from build123d import *
from OCP.BRepFilletAPI import BRepFilletAPI_MakeChamfer

# Parameters (mm, degrees)
EXTRUDE_1_DEPTH                     = 8.5
SKETCH_4_W                          = 0.7
SKETCH_4_H                          = 0.7
CUT_EXTRUDE_1_DEPTH                 = 8.2
CHAMFER_3_SIZE                      = 0.4
SKETCH_2_W                          = 0.4
SKETCH_2_H                          = 0.6
EXTRUDE_2_DEPTH                     = 3
CHAMFER_2_SIZE                      = 0.5
CHAMFER_2_SIZE2                     = 0.106278281
PATTERN_LINEAR_1_COUNT              = 3
PATTERN_LINEAR_1_PITCH              = 2.54
PATTERN_LINEAR_1_COUNT_DIR2         = 2
PATTERN_LINEAR_1_PITCH_DIR2         = 2.54
CHAMFER_3_OF_PATTERN_LINEAR_1_SIZE  = 0.4
CHAMFER_2_OF_PATTERN_LINEAR_1_SIZE  = 0.5
CHAMFER_2_OF_PATTERN_LINEAR_1_SIZE2 = 0.106278281


with BuildPart() as part:
    # Эскиз1 → Бобышка-Вытянуть1 (new body)
    with BuildSketch(Plane(origin=(0, 0, 0), x_dir=(-1, 0, 0), z_dir=(0, 1, 0))):
        Polygon((-1.27, 1.52), (1.27, 1.52), (3.81, 1.52), (3.81, -1.52), (3.81, -6.6), (-1.27, -6.6), (-1.27, -1.52), align=None)
    extrude(amount=EXTRUDE_1_DEPTH)

    # Эскиз4 → Вырез-Вытянуть1 (cut)
    with BuildSketch(Plane(origin=(0, 8.5, 0), x_dir=(1, 0, 0), z_dir=(0, 1, 0))):
        Rectangle(SKETCH_4_W, SKETCH_4_H)
    cut_extrude_1 = extrude(amount=-CUT_EXTRUDE_1_DEPTH, mode=Mode.SUBTRACT)

    # Фаска3
    chamfer_3_edges = [part.edges().sort_by_distance(p)[0] for p in [
        (-0.35, 8.5, 0),
        (0, 8.5, 0.35),
        (0.35, 8.5, 0),
        (0, 8.5, -0.35),
    ]]
    chamfer(chamfer_3_edges, length=CHAMFER_3_SIZE)

    # Эскиз2 → Бобышка-Вытянуть2 (add)
    with BuildSketch(Plane(origin=(0, 0, 0), x_dir=(-1, 0, 0), z_dir=(0, 1, 0))):
        Rectangle(SKETCH_2_W, SKETCH_2_H)
    extrude_2 = extrude(amount=-EXTRUDE_2_DEPTH)

    # Фаска2: one chamfer whose edges measure the first distance from different faces: ONE call of the kernel's chamfer builder (chamfer() names one face for all edges)
    chamfer_2_edges_1 = [part.edges().sort_by_distance(p)[0] for p in [
        (-0.2, -3, 0),
    ]]
    chamfer_2_side_1 = [part.faces().sort_by_distance(p)[0] for p in [
        (-0.2, -1.5, 0),
    ]]
    chamfer_2_edges_2 = [part.edges().sort_by_distance(p)[0] for p in [
        (0.2, -3, 0),
    ]]
    chamfer_2_side_2 = [part.faces().sort_by_distance(p)[0] for p in [
        (0.2, -1.5, 0),
    ]]
    chamfer_2 = BRepFilletAPI_MakeChamfer(part.part.solid().wrapped)
    for e in chamfer_2_edges_1:
        chamfer_2.Add(CHAMFER_2_SIZE, CHAMFER_2_SIZE2, e.wrapped, chamfer_2_side_1[0].wrapped)  # the first distance lies on this face
    for e in chamfer_2_edges_2:
        chamfer_2.Add(CHAMFER_2_SIZE, CHAMFER_2_SIZE2, e.wrapped, chamfer_2_side_2[0].wrapped)  # the first distance lies on this face
    add(Compound.cast(chamfer_2.Shape()), mode=Mode.REPLACE)

    # Линейный массив1: Вырез-Вытянуть1, Extrude 2 3 × 2
    with Locations(*[(-j * PATTERN_LINEAR_1_PITCH_DIR2, 0, -i * PATTERN_LINEAR_1_PITCH) for i in range(PATTERN_LINEAR_1_COUNT) for j in range(PATTERN_LINEAR_1_COUNT_DIR2) if (i, j) != (0, 0)]):
        add(cut_extrude_1, mode=Mode.SUBTRACT)
        add(extrude_2)

    # Фаска3 of Линейный массив1
    chamfer_3_of_pattern_linear_1_edges = [part.edges().sort_by_distance(p)[0] for p in [
        (-2.89, 8.5, 0),
        (-2.54, 8.5, 0.35),
        (-2.19, 8.5, 0),
        (-2.54, 8.5, -0.35),
        (-0.35, 8.5, -2.54),
        (0, 8.5, -2.19),
        (0.35, 8.5, -2.54),
        (0, 8.5, -2.89),
        (-2.89, 8.5, -2.54),
        (-2.54, 8.5, -2.19),
        (-2.19, 8.5, -2.54),
        (-2.54, 8.5, -2.89),
        (-0.35, 8.5, -5.08),
        (0, 8.5, -4.73),
        (0.35, 8.5, -5.08),
        (0, 8.5, -5.43),
        (-2.89, 8.5, -5.08),
        (-2.54, 8.5, -4.73),
        (-2.19, 8.5, -5.08),
        (-2.54, 8.5, -5.43),
    ]]
    chamfer(chamfer_3_of_pattern_linear_1_edges, length=CHAMFER_3_OF_PATTERN_LINEAR_1_SIZE)

    # Фаска2 of Линейный массив1: one chamfer whose edges measure the first distance from different faces: ONE call of the kernel's chamfer builder (chamfer() names one face for all edges)
    chamfer_2_of_pattern_linear_1_edges_1 = [part.edges().sort_by_distance(p)[0] for p in [
        (-2.74, -3, 0),
    ]]
    chamfer_2_of_pattern_linear_1_side_1 = [part.faces().sort_by_distance(p)[0] for p in [
        (-2.74, -1.5, 0),
    ]]
    chamfer_2_of_pattern_linear_1_edges_2 = [part.edges().sort_by_distance(p)[0] for p in [
        (-2.34, -3, 0),
    ]]
    chamfer_2_of_pattern_linear_1_side_2 = [part.faces().sort_by_distance(p)[0] for p in [
        (-2.34, -1.5, 0),
    ]]
    chamfer_2_of_pattern_linear_1_edges_3 = [part.edges().sort_by_distance(p)[0] for p in [
        (-0.2, -3, -2.54),
    ]]
    chamfer_2_of_pattern_linear_1_side_3 = [part.faces().sort_by_distance(p)[0] for p in [
        (-0.2, -1.5, -2.54),
    ]]
    chamfer_2_of_pattern_linear_1_edges_4 = [part.edges().sort_by_distance(p)[0] for p in [
        (0.2, -3, -2.54),
    ]]
    chamfer_2_of_pattern_linear_1_side_4 = [part.faces().sort_by_distance(p)[0] for p in [
        (0.2, -1.5, -2.54),
    ]]
    chamfer_2_of_pattern_linear_1_edges_5 = [part.edges().sort_by_distance(p)[0] for p in [
        (-2.74, -3, -2.54),
    ]]
    chamfer_2_of_pattern_linear_1_side_5 = [part.faces().sort_by_distance(p)[0] for p in [
        (-2.74, -1.5, -2.54),
    ]]
    chamfer_2_of_pattern_linear_1_edges_6 = [part.edges().sort_by_distance(p)[0] for p in [
        (-2.34, -3, -2.54),
    ]]
    chamfer_2_of_pattern_linear_1_side_6 = [part.faces().sort_by_distance(p)[0] for p in [
        (-2.34, -1.5, -2.54),
    ]]
    chamfer_2_of_pattern_linear_1_edges_7 = [part.edges().sort_by_distance(p)[0] for p in [
        (-0.2, -3, -5.08),
    ]]
    chamfer_2_of_pattern_linear_1_side_7 = [part.faces().sort_by_distance(p)[0] for p in [
        (-0.2, -1.5, -5.08),
    ]]
    chamfer_2_of_pattern_linear_1_edges_8 = [part.edges().sort_by_distance(p)[0] for p in [
        (0.2, -3, -5.08),
    ]]
    chamfer_2_of_pattern_linear_1_side_8 = [part.faces().sort_by_distance(p)[0] for p in [
        (0.2, -1.5, -5.08),
    ]]
    chamfer_2_of_pattern_linear_1_edges_9 = [part.edges().sort_by_distance(p)[0] for p in [
        (-2.74, -3, -5.08),
    ]]
    chamfer_2_of_pattern_linear_1_side_9 = [part.faces().sort_by_distance(p)[0] for p in [
        (-2.74, -1.5, -5.08),
    ]]
    chamfer_2_of_pattern_linear_1_edges_10 = [part.edges().sort_by_distance(p)[0] for p in [
        (-2.34, -3, -5.08),
    ]]
    chamfer_2_of_pattern_linear_1_side_10 = [part.faces().sort_by_distance(p)[0] for p in [
        (-2.34, -1.5, -5.08),
    ]]
    chamfer_2_of_pattern_linear_1 = BRepFilletAPI_MakeChamfer(part.part.solid().wrapped)
    for e in chamfer_2_of_pattern_linear_1_edges_1:
        chamfer_2_of_pattern_linear_1.Add(CHAMFER_2_OF_PATTERN_LINEAR_1_SIZE, CHAMFER_2_OF_PATTERN_LINEAR_1_SIZE2, e.wrapped, chamfer_2_of_pattern_linear_1_side_1[0].wrapped)  # the first distance lies on this face
    for e in chamfer_2_of_pattern_linear_1_edges_2:
        chamfer_2_of_pattern_linear_1.Add(CHAMFER_2_OF_PATTERN_LINEAR_1_SIZE, CHAMFER_2_OF_PATTERN_LINEAR_1_SIZE2, e.wrapped, chamfer_2_of_pattern_linear_1_side_2[0].wrapped)  # the first distance lies on this face
    for e in chamfer_2_of_pattern_linear_1_edges_3:
        chamfer_2_of_pattern_linear_1.Add(CHAMFER_2_OF_PATTERN_LINEAR_1_SIZE, CHAMFER_2_OF_PATTERN_LINEAR_1_SIZE2, e.wrapped, chamfer_2_of_pattern_linear_1_side_3[0].wrapped)  # the first distance lies on this face
    for e in chamfer_2_of_pattern_linear_1_edges_4:
        chamfer_2_of_pattern_linear_1.Add(CHAMFER_2_OF_PATTERN_LINEAR_1_SIZE, CHAMFER_2_OF_PATTERN_LINEAR_1_SIZE2, e.wrapped, chamfer_2_of_pattern_linear_1_side_4[0].wrapped)  # the first distance lies on this face
    for e in chamfer_2_of_pattern_linear_1_edges_5:
        chamfer_2_of_pattern_linear_1.Add(CHAMFER_2_OF_PATTERN_LINEAR_1_SIZE, CHAMFER_2_OF_PATTERN_LINEAR_1_SIZE2, e.wrapped, chamfer_2_of_pattern_linear_1_side_5[0].wrapped)  # the first distance lies on this face
    for e in chamfer_2_of_pattern_linear_1_edges_6:
        chamfer_2_of_pattern_linear_1.Add(CHAMFER_2_OF_PATTERN_LINEAR_1_SIZE, CHAMFER_2_OF_PATTERN_LINEAR_1_SIZE2, e.wrapped, chamfer_2_of_pattern_linear_1_side_6[0].wrapped)  # the first distance lies on this face
    for e in chamfer_2_of_pattern_linear_1_edges_7:
        chamfer_2_of_pattern_linear_1.Add(CHAMFER_2_OF_PATTERN_LINEAR_1_SIZE, CHAMFER_2_OF_PATTERN_LINEAR_1_SIZE2, e.wrapped, chamfer_2_of_pattern_linear_1_side_7[0].wrapped)  # the first distance lies on this face
    for e in chamfer_2_of_pattern_linear_1_edges_8:
        chamfer_2_of_pattern_linear_1.Add(CHAMFER_2_OF_PATTERN_LINEAR_1_SIZE, CHAMFER_2_OF_PATTERN_LINEAR_1_SIZE2, e.wrapped, chamfer_2_of_pattern_linear_1_side_8[0].wrapped)  # the first distance lies on this face
    for e in chamfer_2_of_pattern_linear_1_edges_9:
        chamfer_2_of_pattern_linear_1.Add(CHAMFER_2_OF_PATTERN_LINEAR_1_SIZE, CHAMFER_2_OF_PATTERN_LINEAR_1_SIZE2, e.wrapped, chamfer_2_of_pattern_linear_1_side_9[0].wrapped)  # the first distance lies on this face
    for e in chamfer_2_of_pattern_linear_1_edges_10:
        chamfer_2_of_pattern_linear_1.Add(CHAMFER_2_OF_PATTERN_LINEAR_1_SIZE, CHAMFER_2_OF_PATTERN_LINEAR_1_SIZE2, e.wrapped, chamfer_2_of_pattern_linear_1_side_10[0].wrapped)  # the first distance lies on this face
    add(Compound.cast(chamfer_2_of_pattern_linear_1.Shape()), mode=Mode.REPLACE)


solid = part.part
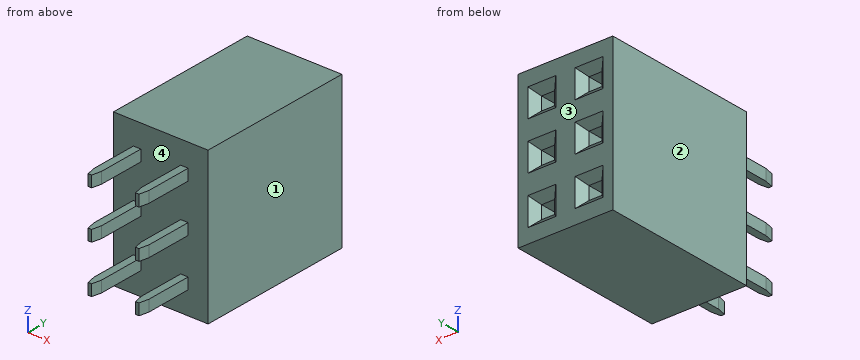
Geometry check sheet. Reference: the model listing, model coordinates, mm. Face numbers are marked on the shaded views. Give positions to 0.01 mm unless a question says otherwise; leave off trailing zeros. Loops run counter-clockwise (first coordinate to the right, second up) from the corner with the lowest first, then second, coordinate; pieces in that order, holes last.
(1) Section check B-B on y = 1. Record the cut outline in (x, z), then the cut area to 3 significant figures.
From the geometry:
outline: (-3.81, -6.6) - (1.27, -6.6) - (1.27, 1.52) - (-3.81, 1.52) - close; hole (-2.89, -5.43) - (-2.19, -5.43) - (-2.19, -4.73) - (-2.89, -4.73) - close; hole (-2.89, -2.89) - (-2.19, -2.89) - (-2.19, -2.19) - (-2.89, -2.19) - close; hole (-2.89, -0.35) - (-2.19, -0.35) - (-2.19, 0.35) - (-2.89, 0.35) - close; hole (-0.35, -5.43) - (0.35, -5.43) - (0.35, -4.73) - (-0.35, -4.73) - close; hole (-0.35, -2.89) - (0.35, -2.89) - (0.35, -2.19) - (-0.35, -2.19) - close; hole (-0.35, -0.35) - (0.35, -0.35) - (0.35, 0.35) - (-0.35, 0.35) - close
area: 38.3 mm2
(2) Section check D-D on x = -0.9. Record the cut outline in (y, z), then the cut area to 3 significant figures.
From the geometry:
outline: (0, -6.6) - (8.5, -6.6) - (8.5, 1.52) - (0, 1.52) - close
area: 69.0 mm2
(3) Thickness scan on L1, parallel to Z at x = -2.4, y = 7; L2, parallel to X at y = 3.75, z = -2.75; L3, parallel to Z at x = -2.55, y = -1. Record the ranges inside material, lowest first.
From the geometry:
L1: z = -6.6 to -5.43, -4.73 to -2.89, -2.19 to -0.35, 0.35 to 1.52
L2: x = -3.81 to -2.89, -2.19 to -0.35, 0.35 to 1.27
L3: z = -5.38 to -4.78, -2.84 to -2.24, -0.3 to 0.3
(4) Section check A-A on y = -2. Record the cut outline in (x, z).
From the geometry:
outline: (-2.74, -5.38) - (-2.34, -5.38) - (-2.34, -4.78) - (-2.74, -4.78) - close; (-2.74, -2.84) - (-2.34, -2.84) - (-2.34, -2.24) - (-2.74, -2.24) - close; (-2.74, -0.3) - (-2.34, -0.3) - (-2.34, 0.3) - (-2.74, 0.3) - close; (-0.2, -5.38) - (0.2, -5.38) - (0.2, -4.78) - (-0.2, -4.78) - close; (-0.2, -2.84) - (0.2, -2.84) - (0.2, -2.24) - (-0.2, -2.24) - close; (-0.2, -0.3) - (0.2, -0.3) - (0.2, 0.3) - (-0.2, 0.3) - close
(5) Section check C-C on z = 0. Record the cut outline in (x, y).
From the geometry:
outline: (-3.81, 0) - (-2.74, 0) - (-2.74, -2.5) - (-2.63, -3) - (-2.45, -3) - (-2.34, -2.5) - (-2.34, 0) - (-0.2, 0) - (-0.2, -2.5) - (-0.09, -3) - (0.09, -3) - (0.2, -2.5) - (0.2, 0) - (1.27, 0) - (1.27, 8.5) - (0.75, 8.5) - (0.35, 8.1) - (0.35, 0.3) - (-0.35, 0.3) - (-0.35, 8.1) - (-0.75, 8.5) - (-1.79, 8.5) - (-2.19, 8.1) - (-2.19, 0.3) - (-2.89, 0.3) - (-2.89, 8.1) - (-3.29, 8.5) - (-3.81, 8.5) - close
(6) Depth check by flat-ended pin: pin 1 Ø0.8 at (x, z) = (0, -5) entering from +Y; pin 2 Ø0.5 at (y, z) = (-1, 0) entering from +X; pin 3 Ø1.5 at (x, z) = (-1.5, -4) entering from -Y. Enter the tip coordinate at first touch or a pass-through.
From the geometry:
pin 1: stops at y = 8.23
pin 2: stops at x = 0.2
pin 3: stops at y = 0
(7) Release check for a two-part mould opening along X. For the marked faces 1, 2, 3 and 4 record: released by +X, released by -X, zero draft, split by the parting line, or undercut.
From the geometry:
face 1: released by +X
face 2: released by -X
face 3: zero draft
face 4: undercut
